Here's the drawing with two shaded views (mm, measured from the low corner). I have some questions. A direction names the side the tool comes from. Coordinates: 2 decimals unless noted, no trailing zeros. Write each loop counter-clockwise with the first axis right and the second up, starting at its lowest first coordinate (ties: lowest second). Pieces come first, ordered by that corner, then holes. Notation, with made-up numbers: (-29, -14) -> (10, -14) arc R16 ccw to (10, -1) -> close; hole circle Ø6 at (29.5, 4). An arc over 180 degrees is marked (long way). Use one line per item in the form item = value.
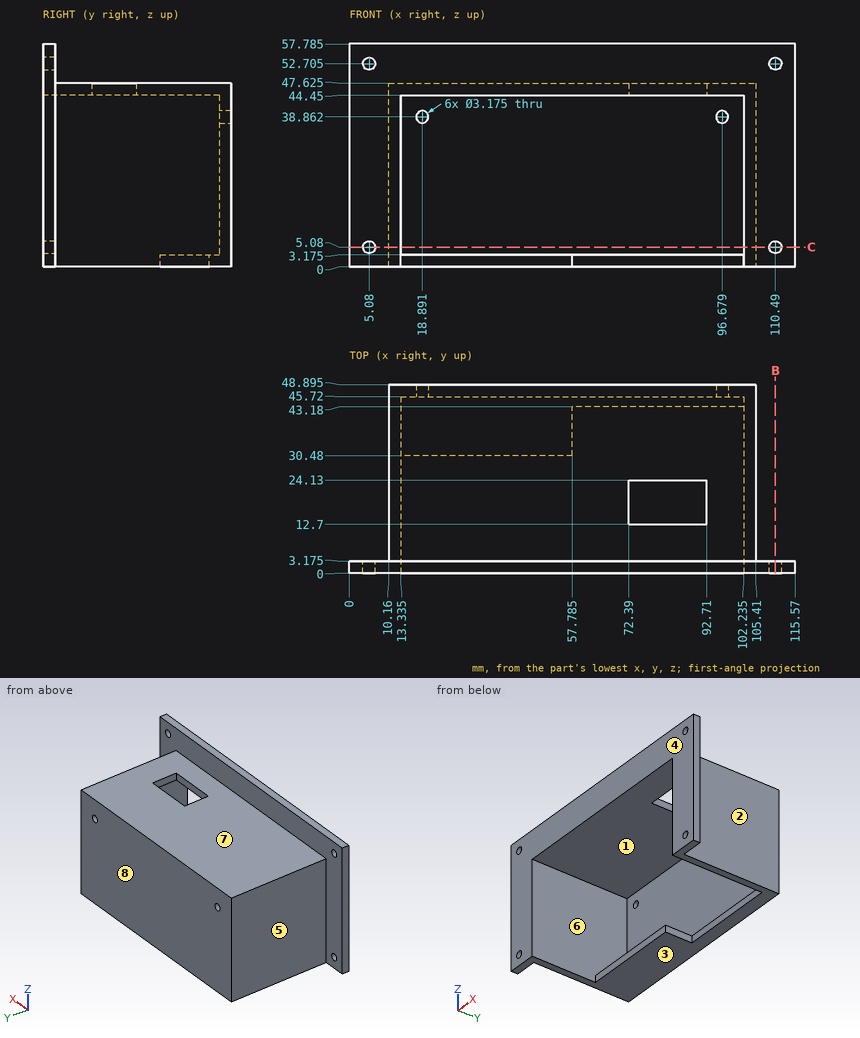
Q1. Suppose I cut it at B-B (x = 110.49). Write out the boundary of the cut face in (y, z) (1 decimal).
Return value:
outline = (0, 0) -> (3.2, 0) -> (3.2, 3.5) -> (0, 3.5) -> close; (0, 6.7) -> (3.2, 6.7) -> (3.2, 51.1) -> (0, 51.1) -> close; (0, 54.3) -> (3.2, 54.3) -> (3.2, 57.8) -> (0, 57.8) -> close
Q2. If I drill on line 1 (X direction, y = 1, z = 5) (1 decimal); line 2 (X direction, y = 27, z = 38) (1 decimal); line 3 (X direction, y = 3, z = 7.5) (1 decimal), over which ranges is the centre line in solid material (lowest first)? Write a range as from..to.
Return value:
line_1 = 0..3.5, 6.7..13.3, 102.2..108.9, 112.1..115.6
line_2 = 10.2..13.3, 102.2..105.4
line_3 = 0..13.3, 102.2..115.6
Q3. Will these pins go through, and if not, where does the flat tip stop? pin 1 (22 mm diameter, centred on y = 23, z = 19, fed in from -X); pin 2 (5 mm diameter, centred on x = 84.5, y = 12.5, fed in from -Z); pin 3 (23 mm diameter, centred on x = 79, y = 28.5, fed in from +Z) (3 decimals).
Return value:
pin_1 = 10.16
pin_2 = 44.45
pin_3 = 47.625
Q4. Suppose I cut it at C-C (z = 5.08). Write out the boundary of the cut face in (x, y) (1 decimal).
Return value:
outline = (0, 0) -> (3.5, 0) -> (3.5, 3.2) -> (0, 3.2) -> close; (6.7, 0) -> (13.3, 0) -> (13.3, 45.7) -> (102.2, 45.7) -> (102.2, 0) -> (108.9, 0) -> (108.9, 3.2) -> (105.4, 3.2) -> (105.4, 48.9) -> (10.2, 48.9) -> (10.2, 3.2) -> (6.7, 3.2) -> close; (112.1, 0) -> (115.6, 0) -> (115.6, 3.2) -> (112.1, 3.2) -> close
Q5. Thinking about a two-plate mould opening in Z: for the marked faces 6, 7 and 8, which applies, released by +Z, released by -Z, zero draft, split by the parting line, or undercut?
Return value:
face_6 = undercut
face_7 = released by +Z
face_8 = zero draft
Q6. For the marked faces 1, 2, 3, 4 and 5, which set-ups out of +Z, -Z, +X, -X, +Y, -Y let a thin tool reach every point of the face, with its end or its side?
Return value:
face_1 = -Y
face_2 = +Z, -Z, +X, +Y
face_3 = -Z, +X, -X, +Y, -Y
face_4 = +Z, -Z, +X, -X, -Y
face_5 = +Z, -Z, -X, +Y
